from build123d import *

# Parameters (mm, degrees)
F0_W     = 101.6
F0_H     = 101.6
F1_DEPTH = 101.6
F2_R     = 25.4
F3_DEPTH = 101.6
F4_W     = 50.8
F4_H     = 50.8
F5_DEPTH = 25.4
F8_R     = 6.35


with BuildPart() as f1:
    # F0 (on Top) → F1 (new body)
    with BuildSketch(Plane.XY):
        Rectangle(F0_W, F0_H)
    extrude(amount=F1_DEPTH)

    # F2 (on face) → F3 (join)
    with BuildSketch(Plane.XY.offset(101.6)):
        Circle(F2_R)
    extrude(amount=F3_DEPTH)

    # F4 (on face) → F5 (cut)
    with BuildSketch(Plane.XZ.offset(50.8)):
        with Locations((0, 50.8)):
            Rectangle(F4_W, F4_H)
    extrude(amount=-F5_DEPTH, mode=Mode.SUBTRACT)

    # F6 (on face) → F7 (revolve)
    with BuildSketch(Plane.XY.offset(203.2)):
        with BuildLine():
            Line((0, -25.4), (0, -38.1))
            ThreePointArc((0, -38.1), (38.1, 0), (0, 38.1))
            Line((0, 38.1), (0, 25.4))
            ThreePointArc((0, 25.4), (17.9605122421, 17.9605122421), (25.4, 0))
            ThreePointArc((25.4, 0), (17.9605122421, -17.9605122421), (0, -25.4))
        make_face()
    revolve(axis=Axis((0, 0, 203.2), (0, -1, 0)))

    # F8
    f8_edges = [f1.edges().sort_by_distance(p)[0] for p in [
        (0, -50.8, 101.6),
        (-50.8, 0, 101.6),
        (0, 50.8, 101.6),
        (50.8, 0, 101.6),
        (50.8, -50.8, 50.8),
        (-50.8, -50.8, 50.8),
        (50.8, 0, 0),
        (0, -50.8, 0),
        (50.8, 50.8, 50.8),
        (-25.4, 0, 174.801937),
        (-25.4, 0, 101.6),
        (25.4, 0, 138.200968),
        (-50.8, 50.8, 50.8),
        (-50.8, 0, 0),
        (0, 50.8, 0),
    ]]
    fillet(f8_edges, radius=F8_R)


solid = f1.part
Model file for the job. Use its own axes, mm. A direction names the side the tool comes from. Give positions to 0.01 mm unless a question says otherwise; leave off trailing zeros. Write each loop counter-clockwise with the first axis right and the second up, starting at its lowest first coordinate (ties: lowest second). Pieces come first, ordered by that corner, then holes. Notation, with made-up numbers: (19, -31) - (29, -31) arc R34 ccw to (29, 5) - close; hole circle Ø11 at (85, -36). An arc over 180 degrees is marked (long way). Answer as CSV lines item,"result".
1. Band-saw the part on A-A (y = 35.5). Write the cut outline in (x, z).
Responses:
outline,"(-50.8, 6.35) arc R6.35 ccw to (-44.45, 0) - (44.45, 0) arc R6.35 ccw to (50.8, 6.35) - (50.8, 95.25) arc R6.35 ccw to (44.45, 101.6) - (-44.45, 101.6) arc R6.35 ccw to (-50.8, 95.25) - close; circle Ø27.67 at (0, 203.2)"
2. Two-plate mould, pull along X, no slides. Class faces 1 (the face through (-48.89, 0.62, 99.79)), 2 (the face through (-1, 1, 0)), 3 (the face through (-25.4, -38, 50)): +X half, -X half, draft (parallel to the pull), parting line (faces both ways), or undercut.
Responses:
face 1,"-X half"
face 2,"draft"
face 3,"undercut"
3. Band-saw the part on C-C (z = 179). Write the cut outline in (x, y).
Responses:
outline,"circle Ø58.85 at (0, 0)"
4. 3-axis set-ups, long thin cutter, end or side, ignore diameter. For faces 4 (the face through (48.89, 48.99, 51.42)), 5 (the face through (25.4, -38, 50)), 6 (the face through (-11, 30, 101.6)): which of +Z, -Z, +X, -X, +Y, -Y reach the whole face in a straight line?
Responses:
face 4,"+Z, -Z, +X, +Y"
face 5,"-Y"
face 6,"none"
5. Drill centre lines: L1, parallel to X at y = -36, z = 60.5; L2, parallel to Z at x = 19, y = -29; L3, parallel to Z at x = -23.5, y = 37.5. Where is each one in solid material? Low to high. Write a range as [from, to].
Responses:
L1,"x = [-50.8, -25.4], [25.4, 50.8]"
L2,"z = [0, 25.4], [76.2, 101.6], [187.4, 219]"
L3,"z = [0, 101.6]"
6. Pin check, flat tips, straight feed: pin 1 (8 mm diameter, centred on x = -25, z = 26, fed in from -Y); pin 2 (12.5 mm diameter, centred on x = -4, y = -37, fed in from +Z); pin 3 (8 mm diameter, centred on x = 17.5, y = 23.5, fed in from +Z); pin 4 (2 mm diameter, centred on x = -13.5, z = 130.5, fed in from -Y). Stop position of each tip, or through.
Responses:
pin 1,"stops at y = -50.8"
pin 2,"stops at z = 225.4"
pin 3,"stops at z = 231.69"
pin 4,"stops at y = -22.11"
7. Band-saw the part on B-B (z = 221.5). Write the cut outline in (x, y).
Responses:
outline,"circle Ø66.83 at (0, 0); hole circle Ø35.23 at (0, 0)"
